Geometry check sheet. Reference: the model listing, model coordinates, mm. A direction names the side the tool comes from. Round coordinates to 2 decimals unless told otherwise and drop trailing zeros. Write each loop counter-clockwise with the first axis right and the second up, starting at its lowest first coordinate (ties: lowest second). Pieces come first, ordered by that corner, then holes.
Item 1: Depth check by flat-ended pin: P1, Ø16, axis at x = -105.5, z = -12.5, coming from the +Y side. Enter the tip coordinate at first touch or a pass-through.
Item 2: Scan lines: probe 1 along Z at (x, y) = (26, 6); probe 2 along X at (y, z) = (0.5, -22); probe 3 along Z at (x, y) = (72, 24). Record each from-to range of solid material in increasing order.
Item 3: Draft check along Z on faces 1 (the face through (72.26, 24.58, -86.5)), 2 (the face through (125.57, 9.82, -85.72)), 3 (the face through (109.299, -1.146, -69.363)). Enter one of: pulls with the +Z half, pulls with the -Z half, needs draft (parallel to the pull), parting line crosses it, or undercut.
Item 4: Access from +Z, -Z, +X, -X, +Y, -Y to the whole of each face (thin tool, end or side, straight path). Record for faces 4 (the face through (-123.48, 11.34, -83.57)), 5 (the face through (-126, 23, -27)), 6 (the face through (-109.363, -1.146, -69.299)), 7 (the face through (2, 11, -85.4)), 8 (the face through (125.72, 9.82, 85.57)).
Item 5: Cross-section at C-C (y = 4.5). Enter the section's corners in (x, z).
from build123d import *

# Parameters (mm, degrees)
BOSS_EXTRUDE1_DEPTH = 23
BOSS_EXTRUDE2_START = 3
SKETCH2_W           = 218.8
SKETCH2_H           = 138.8
BOSS_EXTRUDE2_DEPTH = 3
FILLET1_R           = 3
CHAMFER1_SIZE       = 3
BOSS_EXTRUDE4_DEPTH = 5
CHAMFER2_SIZE       = 3
CUT_EXTRUDE1_DEPTH  = 5


# Read off the part's stored shape, not the designer's step: Mirror1
with BuildPart() as part:
    # Sketch1 → Boss-Extrude1 (new body)
    with BuildSketch(Plane(origin=(0, 0, 0), x_dir=(1, 0, 0), z_dir=(0, 1, 0))):
        with BuildLine():
            Line((119, 88.4), (-119, 88.4))
            ThreePointArc((-119, 88.4), (-125.646803743, 85.646803743), (-128.4, 79))
            Line((-128.4, 79), (-128.4, -79))
            ThreePointArc((-128.4, -79), (-125.646803743, -85.646803743), (-119, -88.4))
            Line((-119, -88.4), (119, -88.4))
            ThreePointArc((119, -88.4), (125.646803743, -85.646803743), (128.4, -79))
            Line((128.4, -79), (128.4, 79))
            ThreePointArc((128.4, 79), (125.646803743, 85.646803743), (119, 88.4))
        make_face()
        with BuildLine():
            Line((-125.4, 79), (-125.4, -79))
            ThreePointArc((-125.4, -79), (-123.5254834, -83.5254834), (-119, -85.4))
            Line((-119, -85.4), (119, -85.4))
            ThreePointArc((119, -85.4), (123.5254834, -83.5254834), (125.4, -79))
            Line((125.4, -79), (125.4, 79))
            ThreePointArc((125.4, 79), (123.5254834, 83.5254834), (119, 85.4))
            Line((119, 85.4), (-119, 85.4))
            ThreePointArc((-119, 85.4), (-123.5254834, 83.5254834), (-125.4, 79))
        make_face(mode=Mode.SUBTRACT)
    extrude(amount=BOSS_EXTRUDE1_DEPTH)

    # Sketch2 → Boss-Extrude2 (add)
    with BuildSketch(Plane.XZ.offset(BOSS_EXTRUDE2_START)):
        with BuildLine():
            Line((128.4, -79), (128.4, 79))
            ThreePointArc((128.4, 79), (125.646803743, 85.646803743), (119, 88.4))
            Line((119, 88.4), (-119, 88.4))
            ThreePointArc((-119, 88.4), (-125.646803743, 85.646803743), (-128.4, 79))
            Line((-128.4, 79), (-128.4, -79))
            ThreePointArc((-128.4, -79), (-125.646803743, -85.646803743), (-119, -88.4))
            Line((-119, -88.4), (119, -88.4))
            ThreePointArc((119, -88.4), (125.646803743, -85.646803743), (128.4, -79))
        make_face()
        Rectangle(SKETCH2_W, SKETCH2_H, mode=Mode.SUBTRACT)
    extrude(amount=-BOSS_EXTRUDE2_DEPTH)

    # Fillet1
    fillet1_edges = [part.edges().sort_by_distance(p)[0] for p in [
        (109.4, -1.5, 69.4),
        (-109.4, -1.5, 69.4),
        (-109.4, -1.5, -69.4),
        (109.4, -1.5, -69.4),
    ]]
    fillet(fillet1_edges, radius=FILLET1_R)

    # Chamfer1
    chamfer1_edges = [part.edges().sort_by_distance(p)[0] for p in [
        (109.4, -3, 0),
        (108.521320344, -3, 68.521320344),
        (108.521320344, -3, -68.521320344),
        (0, -3, 69.4),
        (0, -3, -69.4),
        (-108.521320344, -3, 68.521320344),
        (-108.521320344, -3, -68.521320344),
        (-109.4, -3, 0),
    ]]
    chamfer(chamfer1_edges, length=CHAMFER1_SIZE - 0.0001)  # a hair under: the kernel refuses the full size

    # Sketch4 → Boss-Extrude4 (add)
    with BuildSketch(Plane.XY.offset(88.4)):
        Polygon((75, 23), (-75, 23), (-68.07179677, 27), (68.07179677, 27), align=None)
    extrude(amount=-BOSS_EXTRUDE4_DEPTH)

    # Chamfer2
    chamfer2_edges = [part.edges().sort_by_distance(p)[0] for p in [
        (0, 27, 83.4),
    ]]
    chamfer(chamfer2_edges, length=CHAMFER2_SIZE)

    # Sketch5 → Cut-Extrude1 (cut)
    with BuildSketch(Plane(origin=(0, 27, 0), x_dir=(1, 0, 0), z_dir=(0, 1, 0))):
        with BuildLine():
            Line((-73, -83.4), (-75, -83.4))
            Line((-75, -83.4), (-75, -85.4))
            ThreePointArc((-75, -85.4), (-74.414213562, -83.985786438), (-73, -83.4))
        make_face()
        with BuildLine():
            Line((75, -83.4), (75, -85.4))
            ThreePointArc((75, -85.4), (74.414213562, -83.985786438), (73, -83.4))
            Line((73, -83.4), (75, -83.4))
        make_face()
    extrude(amount=-CUT_EXTRUDE1_DEPTH, mode=Mode.SUBTRACT)

    # Mirror1: part across plane


with BuildPart() as part_1:
    add(part.part)
    add(part.part.mirror(Plane.XY))


solid = part_1.part
Resolved:
1. P1: stops at y = 0
2. probe 1: z = -88.4 to -85.4, 85.4 to 88.4
2. probe 2: x = -128.4 to -125.4, 125.4 to 128.4
2. probe 3: z = -88.4 to -83.4, 83.4 to 88.4
3. face 1: needs draft
3. face 2: pulls with the -Z half
3. face 3: undercut
4. face 4: +Y
4. face 5: +Z, -Z, -X, +Y
4. face 6: -Y
4. face 7: none
4. face 8: +Z, +X, +Y, -Y
5. outline: (-128.4, -79) arc R9.4 ccw to (-119, -88.4) - (119, -88.4) arc R9.4 ccw to (128.4, -79) - (128.4, 79) arc R9.4 ccw to (119, 88.4) - (-119, 88.4) arc R9.4 ccw to (-128.4, 79) - close; hole (-125.4, -79) arc R6.4 ccw to (-119, -85.4) - (119, -85.4) arc R6.4 ccw to (125.4, -79) - (125.4, 79) arc R6.4 ccw to (119, 85.4) - (-119, 85.4) arc R6.4 ccw to (-125.4, 79) - close
